Work out the finished part from the listing and answer in its coordinate system (mm). Face numbers are marked on the shaded views. A direction names the side the tool comes from. Coordinates: 2 decimals unless noted, no trailing zeros. Order: outer loops, then holes, each group sorted by start corner. A loop starts at its lowest first (then second) coordinate and runs counter-clockwise, first axis right, second up. Notation, with made-up numbers: (35.25, -10.75) -> (41.25, -10.75) arc R33 ccw to (41.25, 22.25) -> close; hole circle Ø3 at (-11.75, 40.25). An arc over 180 degrees is marked (long way). Write item = value, one per line. Start each with the question number.
Q1. Straight lines are drawn through the part: L1, parallel to X at y = -0.5, z = 2.5; L2, parallel to Y at x = 20.5, z = 3; L3, parallel to X at y = 8.5, z = 6. For each, find the intervals that lie inside material, in ascending order. Write a range as from..to.
Q2. The part is cut by section B-B, the plane y = -8. Determine the outline of the cut face in (x, z), plus the area to 3 significant figures.
Q3. For a pull along X with two mould halves and no side action, classify the marked faces 1, 2 and 3 as +X half, -X half, draft (parallel to the pull), parting line (faces both ways), or undercut.
Q4. The part is cut by section A-A, the plane x = 26.65. Determine the outline of the cut face in (y, z), plus the area to 3 significant figures.
Q5. Which of the six approach directions +Z, -Z, +X, -X, +Y, -Y give full straight-line access (tool end or side, diameter ignored) to the marked faces 4, 5 and 6?
Q6. Flat-ended cylindrical pins translate along their axes: pin 1 (4 mm diameter, centred on x = 6, z = 6.5, fed in from +Y); pin 2 (1.5 mm diameter, centred on x = -14, z = 4.5, fed in from +Y); pin 3 (5 mm diameter, centred on y = -5, z = 5, fed in from +X). Find the tip coordinate at first contact, or state that the pin passes through.
Q7. The part is cut by section D-D, the plane x = -4. Determine the outline of the cut face in (y, z), plus the area to 3 significant figures.
Q8. The part is cut by section C-C, the plane z = 4. Determine the outline of the cut face in (x, y).
```python
from build123d import *

# Parameters (mm, degrees)
SALIENTE_EXTRUIR1_DEPTH = 10
CROQUIS2_R              = 2
CORTAR_EXTRUIR1_DEPTH   = 10


with BuildPart() as part:
    # Croquis1 → Saliente-Extruir1 (new body)
    with BuildSketch(Plane.XY):
        with BuildLine():
            Line((10.65, 0), (10.65, -15))
            Line((10.65, -15), (40.65, -15))
            Line((40.65, -15), (40.65, -14))
            Line((40.65, -14), (39.65, -14))
            Line((39.65, -14), (11.65, -14))
            Line((11.65, -14), (11.65, 0))
            ThreePointArc((11.65, 0), (0, 11.65), (-11.65, 0))
            Line((-11.65, 0), (-11.65, -14))
            Line((-11.65, -14), (-39.65, -14))
            Line((-39.65, -14), (-40.65, -14))
            Line((-40.65, -14), (-40.65, -15))
            Line((-40.65, -15), (-10.65, -15))
            Line((-10.65, -15), (-10.65, 0))
            ThreePointArc((-10.65, 0), (0, 10.65), (10.65, 0))
        make_face()
    extrude(amount=SALIENTE_EXTRUIR1_DEPTH)

    # Croquis2 → Cortar-Extruir1 (cut)
    with BuildSketch(Plane(origin=(0, -16.507351352, 0), x_dir=(1, 0, 0), z_dir=(0, 1, 0))):
        with Locations(Location((-26.65, -5, 0), (0, 0, 90))):
            Circle(CROQUIS2_R)
        with Locations((26.65, -5)):
            Circle(CROQUIS2_R)
    extrude(amount=CORTAR_EXTRUIR1_DEPTH, mode=Mode.SUBTRACT)


solid = part.part
```
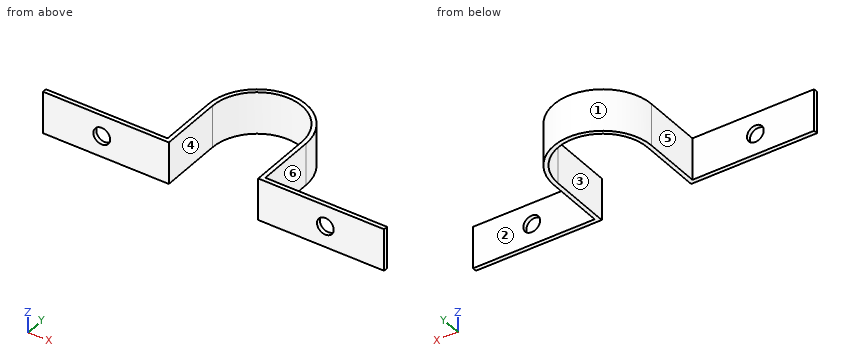
Model answer:
q1.L1 = -11.65..-10.65, 10.65..11.65
q1.L2 = -15..-14
q1.L3 = -7.97..-6.42, 6.42..7.97
q2.outline = (-11.65, 0) -> (-10.65, 0) -> (-10.65, 10) -> (-11.65, 10) -> close; (10.65, 0) -> (11.65, 0) -> (11.65, 10) -> (10.65, 10) -> close
q2.area = 20.0 mm2
q3.face_1 = parting line
q3.face_2 = draft
q3.face_3 = undercut
q4.outline = (-15, 0) -> (-14, 0) -> (-14, 3) -> (-15, 3) -> close; (-15, 7) -> (-14, 7) -> (-14, 10) -> (-15, 10) -> close
q4.area = 6.00 mm2
q5.face_4 = +Z, -Z, -Y
q5.face_5 = +Z, -Z, -X, +Y
q5.face_6 = +Z, -Z, +X, +Y
q6.pin_1 = 10.94
q6.pin_2 = -14
q6.pin_3 = 11.65
q7.outline = (9.87, 0) -> (10.94, 0) -> (10.94, 10) -> (9.87, 10) -> close
q7.area = 10.7 mm2
q8.outline = (-40.65, -15) -> (-28.38, -15) -> (-28.38, -14) -> (-40.65, -14) -> close; (-24.92, -15) -> (-10.65, -15) -> (-10.65, 0) arc R10.65 cw to (10.65, 0) -> (10.65, -15) -> (24.92, -15) -> (24.92, -14) -> (11.65, -14) -> (11.65, 0) arc R11.65 ccw to (-11.65, 0) -> (-11.65, -14) -> (-24.92, -14) -> close; (28.38, -15) -> (40.65, -15) -> (40.65, -14) -> (28.38, -14) -> close
